Design review of the part built by this model. Coordinates are the model's own, in mm. A direction names the side the tool comes from. Give positions to 0.01 mm unless a question says otherwise; leave off trailing zeros. Order: outer loops, then holes, each group sorted by start corner. A loop starts at its lowest first (then second) coordinate and runs counter-clockwise, first axis right, second up. Notation, with made-up numbers: (4.5, -27) -> (24.5, -27) arc R30 cw to (24.5, 5) -> close; hole circle Ø6 at (-15.5, -22). An arc over 180 degrees is marked (long way). Return JSON: item names as keys, results as strings.
```python
from build123d import *

# Parameters (mm, degrees)
SKIZZE1_W                                           = 135.069444444
SKIZZE1_H                                           = 50
AUFSATZ_LINEAR_AUSTRAGEN1_DEPTH                     = 200
STIRNSENKUNG_F_R_M8_SENKSCHRAUBE_KOPF_B_D           = 9
STIRNSENKUNG_F_R_M8_SENKSCHRAUBE_KOPF_B_CBORE_D     = 15
STIRNSENKUNG_F_R_M8_SENKSCHRAUBE_KOPF_B_CBORE_DEPTH = 6.5
SPIEGELN3_COPY_1_D                                  = 9
SPIEGELN3_COPY_1_CBORE_D                            = 15
SPIEGELN3_COPY_1_CBORE_DEPTH                        = 6.5


with BuildPart() as part:
    # Skizze1 → Aufsatz-Linear austragen1 (new body)
    with BuildSketch(Plane.XY):
        Rectangle(SKIZZE1_W, SKIZZE1_H)
    extrude(amount=AUFSATZ_LINEAR_AUSTRAGEN1_DEPTH)

    # Stirnsenkung für M8 Senkschraube (Kopf Button)4 (through all)
    with Locations(Plane(origin=(0, 25, 0), x_dir=(1, 0, 0), z_dir=(0, 1, 0))):
        with Locations((-52.534722222, -185)):
            stirnsenkung_f_r_m8_senkschraube_kopf_b = CounterBoreHole(STIRNSENKUNG_F_R_M8_SENKSCHRAUBE_KOPF_B_D / 2, STIRNSENKUNG_F_R_M8_SENKSCHRAUBE_KOPF_B_CBORE_D / 2, STIRNSENKUNG_F_R_M8_SENKSCHRAUBE_KOPF_B_CBORE_DEPTH)

    # Spiegeln2: Stirnsenkung für M8 Senkschraube (Kopf Button)4 across plane
    add(stirnsenkung_f_r_m8_senkschraube_kopf_b.mirror(Plane(origin=(0, 0, 0), x_dir=(0, 0, 1), z_dir=(1, 0, 0))), mode=Mode.SUBTRACT)

    # Spiegeln3: Stirnsenkung für M8 Senkschraube (Kopf Button)4 across plane
    add(stirnsenkung_f_r_m8_senkschraube_kopf_b.mirror(Plane.XY.offset(100)), mode=Mode.SUBTRACT)

    # Spiegeln3 copy 1 (through all)
    with Locations(Plane(origin=(0, 25, 200), x_dir=(-1, 0, 0), z_dir=(0, 1, 0))):
        with Locations((-52.534722222, -185)):
            CounterBoreHole(SPIEGELN3_COPY_1_D / 2, SPIEGELN3_COPY_1_CBORE_D / 2, SPIEGELN3_COPY_1_CBORE_DEPTH)


solid = part.part
```
Item 1: Add section A-A (z = 15). Give the boundary of the cut face in (x, y).
Result set:
{"outline": "(-67.53, -25) -> (-57.03, -25) -> (-57.03, 18.5) -> (-60.03, 18.5) -> (-60.03, 25) -> (-67.53, 25) -> close; (-48.03, -25) -> (48.03, -25) -> (48.03, 18.5) -> (45.03, 18.5) -> (45.03, 25) -> (-45.03, 25) -> (-45.03, 18.5) -> (-48.03, 18.5) -> close; (57.03, -25) -> (67.53, -25) -> (67.53, 25) -> (60.03, 25) -> (60.03, 18.5) -> (57.03, 18.5) -> close"}
Item 2: Wall thickness on L1, parallel to X at y = 1, z = 185; L2, parallel to X at y = 23, z = 185; L3, parallel to Z at x = -50, y = -13: over which ranges is each line inside the solid? List them lowest first. Write a range as [from, to].
Result set:
{"L1": "x = [-67.53, -57.03], [-48.03, 48.03], [57.03, 67.53]", "L2": "x = [-67.53, -60.03], [-45.03, 45.03], [60.03, 67.53]", "L3": "z = [0, 11.28], [18.72, 181.28], [188.72, 200]"}
Item 3: Machinability: for faces 1 (the face through (-45.38, 21.8, 17.25)), 2 (the face through (-51.6, -3.6, 189.4)), which of the approach directions +Z, -Z, +X, -X, +Y, -Y give a long, thin tool a straight path to every point of the face, cutting with its end or side? Answer none if there is none.
Result set:
{"face 1": "+Y", "face 2": "+Y, -Y"}
Item 4: Mouldability with a two-part tool opening along Z and no side actions: class faces 3 (the face through (53, 18.5, 190)), 4 (the face through (-67.535, 0, 99)), 5 (the face through (-1, 0, 0)) as released by +Z, released by -Z, zero draft, split by the parting line, or undercut.
Result set:
{"face 3": "undercut", "face 4": "zero draft", "face 5": "released by -Z"}
Item 5: For pin 1 (10.5 mm diameter, centred on x = -52.53, z = 185, fed in from +Y); pin 2 (5 mm diameter, centred on x = 45.5, y = -11, fed in from -Z), all flat-tipped, find the tip position at first contact; note any pin that passes through.
Result set:
{"pin 1": "stops at y = 18.5", "pin 2": "stops at z = 0"}
